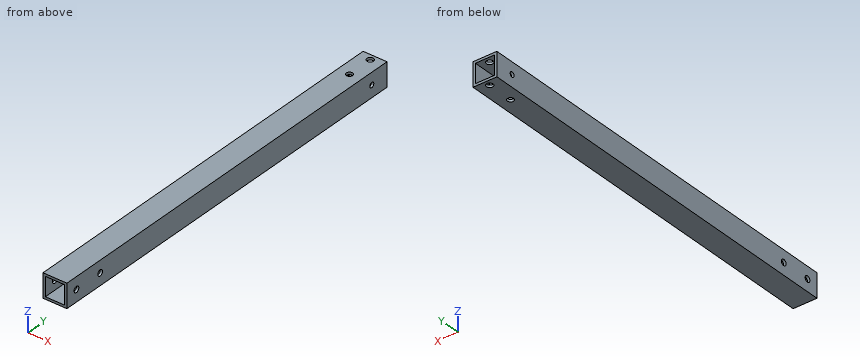
from build123d import *

# Parameters (mm, degrees)
ESBO_O1_W             = 20
ESBO_O1_H             = 20
ESBO_O1_W_2           = 16
ESBO_O1_H_2           = 16
EXTRUS_O_FINA1_DEPTH  = 337
ESBO_O2_R             = 2.5
CORTE_EXTRUS_O1_DEPTH = 21
ESBO_O3_R             = 2.6
ESBO_O3_R_2           = 2.8
CORTE_EXTRUS_O2_DEPTH = 21
ESBO_O4_R             = 2.1
CORTE_EXTRUS_O3_DEPTH = 21


with BuildPart() as part:
    # Esboço1 → Extrusão-Fina1 (new body)
    with BuildSketch(Plane(origin=(0, 0, 0), x_dir=(1, 0, 0), z_dir=(0, 1, 0))):
        with Locations((10, 10)):
            Rectangle(ESBO_O1_W, ESBO_O1_H)
        with Locations((10, 10)):
            Rectangle(ESBO_O1_W_2, ESBO_O1_H_2, mode=Mode.SUBTRACT)
    extrude(amount=EXTRUS_O_FINA1_DEPTH)

    # Esboço2 → Corte-extrusão1 (cut, through all)
    with BuildSketch(Plane.ZY):
        with Locations((-10, 35)):
            Circle(ESBO_O2_R)
        with Locations((-10, 10)):
            Circle(ESBO_O2_R)
    extrude(amount=-CORTE_EXTRUS_O1_DEPTH, mode=Mode.SUBTRACT)

    # Esboço3 → Corte-extrusão2 (cut, through all)
    with BuildSketch(Plane(origin=(0, 0, -20), x_dir=(-1, 0, 0), z_dir=(0, 0, -1))):
        with Locations((-10, 310)):
            Circle(ESBO_O3_R)
        with Locations((-10, 332)):
            Circle(ESBO_O3_R_2)
    extrude(amount=-CORTE_EXTRUS_O2_DEPTH, mode=Mode.SUBTRACT)

    # Esboço4 → Corte-extrusão3 (cut, through all)
    with BuildSketch(Plane(origin=(20, 0, 0), x_dir=(0, 0, -1), z_dir=(1, 0, 0))):
        with Locations((10, 321)):
            Circle(ESBO_O4_R)
    extrude(amount=-CORTE_EXTRUS_O3_DEPTH, mode=Mode.SUBTRACT)


solid = part.part
Could you check a few things on this model? Use its own coordinates, in mm. Give positions to 0.01 mm unless a question says otherwise; leave off trailing zeros. Write each loop counter-clockwise with the first axis right and the second up, starting at its lowest first coordinate (ties: lowest second). Pieces come first, ordered by that corner, then holes. Notation, with made-up numbers: (-19, 1.25) - (25, 1.25) arc R23 cw to (25, 16.25) - close; hole circle Ø11 at (67, 8). An arc over 180 degrees is marked (long way). Use CSV: the item, a comma, the result in double quotes. Start each with the question number.
Item 1: I want a section at A-A, the plane z = -15.25. Please give me the cut outline in (x, y).
Item 2: If I drill on line 1 along Y through (x, z) = (19, -10); line 2 along Y through (x, z) = (10, -0.8); line 3 along Z through (x, y) = (13, 293), over which ranges is the centre line in solid material (lowest first)?
Item 3: I want a section at C-C, the plane y = 332. Please give me the cut outline in (x, z).
Item 4: I want a section at B-B, the plane y = 250. Please give me the cut outline in (x, z), then the cut area to 3 significant figures.
Findings:
1,outline,"(0, 0) - (2, 0) - (2, 337) - (0, 337) - close; (18, 0) - (20, 0) - (20, 337) - (18, 337) - close"
2,line 1,"y = 0 to 7.5, 12.5 to 32.5, 37.5 to 318.9, 323.1 to 337"
2,line 2,"y = 0 to 307.4, 312.6 to 329.2, 334.8 to 337"
2,line 3,"z = -20 to -18, -2 to 0"
3,outline,"(0, -20) - (7.2, -20) - (7.2, -18) - (2, -18) - (2, -2) - (7.2, -2) - (7.2, 0) - (0, 0) - close; (12.8, -20) - (20, -20) - (20, 0) - (12.8, 0) - (12.8, -2) - (18, -2) - (18, -18) - (12.8, -18) - close"
4,outline,"(0, -20) - (20, -20) - (20, 0) - (0, 0) - close; hole (2, -18) - (18, -18) - (18, -2) - (2, -2) - close"
4,area,"144 mm2"
